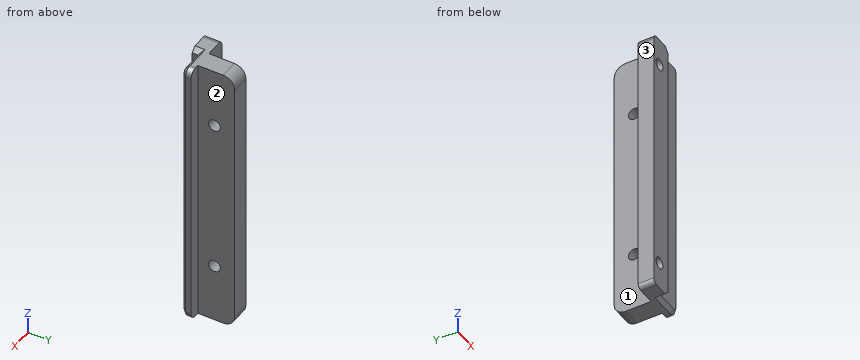
Autodesk Inventor part; units mm, degrees
ref_plane "YZ Plane" through (0, 0, 0) normal (1, 0, 0) x (0, 1, 0)
ref_plane "XZ Plane" through (0, 0, 0) normal (0, 1, 0) x (-1, 0, 0)
ref_plane "XY Plane" through (0, 0, 0) normal (0, 0, 1) x (1, 0, 0)
sketch "Sketch1" plane through (0, 0, 0) normal (0, 0, 1) x (1, 0, 0)
  line L0 (0, 17.3736) -> (0, -2.8956)
  line L1 (-5.334, 0) -> (14.224, 0)
  line L2 (3.81, 1.778) -> (-2.54, 1.778)
  line L3 (-2.54, 1.778) -> (-2.54, 0)
  line L4 (-2.54, 0) -> (3.81, 0)
  line L5 (3.81, 0) -> (3.81, 1.778)
  line L6 (3.81, 1.778) -> (11.43, 1.778)
  line L7 (11.43, 1.778) -> (11.43, 4.318)
  line L8 (11.43, 4.318) -> (-2.54, 4.318)
  line L9 (-2.54, 4.318) -> (-2.54, 1.778)
  line L10 (8.382, 4.318) -> (3.302, 4.318)
  line L11 (3.302, 4.318) -> (3.302, 14.478)
  line L12 (3.302, 14.478) -> (8.382, 14.478)
  line L13 (8.382, 14.478) -> (8.382, 4.318)
  point P0 (0, 0)
  point P1 (0, 0.635)
  dimension "d1" = 2.54
  dimension "d2" = 1.778
  dimension "d25" = 2.54
  dimension "d26" = 10.16
  dimension "d27" = 5.08
  dimension "d49" = 3.302
  dimension "d50" = 2.54
  dimension "d51" = 11.43
  dimension "d52" = 3.81
extrude "Extrusion1" add sketch "Sketch1" along normal mid plane 76.2
sketch "Sketch2" plane through (-2.54, 4.318, 38.1) normal (0, 1, 0) x (1, 0, 0)
  line L0 (13.97, 76.2) -> (13.97, 0)
  line L1 (0, 76.2) -> (13.97, 76.2)
  line L2 (13.97, 0) -> (0, 0)
  line L3 (0, 76.2) -> (0, 0)
  line L4 (16.764, 38.1) -> (-2.794, 38.1)
  point P0 (2.54, 38.1)
  point P1 (2.54, 68.58)
  point P2 (2.54, 38.1)
  point P3 (2.54, 7.62)
  dimension "d6" = 30.48
  dimension "d7" = 30.48
  dimension "d48" = 2.54
hole "Hole1" at (0, 4.318, -30.48) at (0, 4.318, 30.48) direction (0, -1, 0) diameter 3.175 end through all
fillet "Fillet4" radius 1.905 2 edges at (11.43, 3.048, 38.1) (11.43, 3.048, -38.1)
chamfer "Chamfer4" distance 1.016 angle 45 5 edges at (11.43, 1.778, 0) (10.872, 1.778, 37.542) (6.6675, 1.778, 38.1) (10.872, 1.778, -37.542) (6.6675, 1.778, -38.1)
chamfer "Chamfer1" distance 1.27 angle 45 2 edges at (3.81, 0.889, 38.1) (3.81, 0.889, -38.1)
fillet "Fillet3" radius 1.27 2 edges at (-2.54, 2.159, -38.1) (-2.54, 2.159, 38.1)
fillet "Fillet5" radius 3.175 2 edges at (5.842, 14.478, 38.1) (5.842, 14.478, -38.1)
sketch "Sketch3" plane through (8.382, 4.318, 38.1) normal (1, 0, 0) x (0, 0, -1)
  line L0 (74.93, -4.318) -> (1.27, -4.318)
  line L1 (38.1, -7.2136) -> (38.1, 13.0556)
  point P0 (38.1, -4.318)
  point P1 (16.51, 4.572)
  point P2 (59.69, 4.572)
  dimension "d38" = 43.18
  dimension "d39" = 21.59
  dimension "d40" = 8.89
hole "Hole2" at (8.382, 8.89, 21.59) at (8.382, 8.89, -21.59) direction (-1, 0, 0) diameter 3.302 end through all
properties part number "J007812" material "VERO BLACK"
Geometry: final body of the model. Coordinates: model frame, mm. Face numbers are marked on the shaded views. A direction names the side the tool comes from. Round coordinates to 2 decimals unless told otherwise and drop trailing zeros. Write each loop counter-clockwise with the first axis right and the second up, starting at its lowest first coordinate (ties: lowest second). Pieces come first, ordered by that corner, then holes.
Item 1: Section query A-A (y = 8.89). Return loops of the section in (x, z), plus the area to 3 significant figures.
Item 2: Pin query (flat end, axial travel): P1, Ø5, axis at y = 10, z = -8, coming from the +X side; P2, Ø4, axis at x = 0, z = -30.48, coming from the +Y side; P3, Ø5, axis at y = 8, z = -12, coming from the -X side; P4, Ø1.9, axis at x = 0, z = 30.48, coming from the -Y side. Return the tip coordinate at first contact, or that it passes through.
Item 3: Section query C-C (z = -21.59). Return loops of the section in (x, y), plus the area to 3 significant figures.
Item 4: Section query D-D (x = 6). Return loops of the section in (y, z) (3 decimals).
Item 5: Set-up query: the marked faces 1, 2 and 3. Return all of +Z, -Z, +X, -X, +Y, -Y with unobstructed straight access to the full face (end or side cutting, diameter ignored); none if empty.
Item 6: Section query B-B (x = 0). Return loops of the section in (y, z).
Item 7: Material intervals for L1, parallel to Z at x = 0, y = 3; L2, parallel to Z at x = 5.25, y = 8.89; L3, parallel to Y at x = 5.9, z = 21.59, sorted ascending.
Completed:
1. outline: (3.3, -38.1) - (8.38, -38.1) - (8.38, -23.24) - (3.3, -23.24) - close; (3.3, -19.94) - (8.38, -19.94) - (8.38, 19.94) - (3.3, 19.94) - close; (3.3, 23.24) - (8.38, 23.24) - (8.38, 38.1) - (3.3, 38.1) - close
1. area: 354 mm2
2. P1: stops at x = 8.38
2. P2: stops at y = 4.32
2. P3: stops at x = 3.3
2. P4: passes through
3. outline: (-2.54, 0) - (3.81, 0) - (3.81, 1.78) - (10.41, 1.78) - (11.43, 2.79) - (11.43, 4.32) - (8.38, 4.32) - (8.38, 7.24) - (3.3, 7.24) - (3.3, 4.32) - (-2.54, 4.32) - close; (3.3, 10.54) - (8.38, 10.54) - (8.38, 14.48) - (3.3, 14.48) - close
3. area: 81.1 mm2
4. outline: (1.778, -37.084) - (2.794, -38.1) - (11.303, -38.1) arc R3.175 ccw to (14.478, -34.925) - (14.478, 34.925) arc R3.175 ccw to (11.303, 38.1) - (2.794, 38.1) - (1.778, 37.084) - close; hole circle Ø3.302 at (8.89, -21.59); hole circle Ø3.302 at (8.89, 21.59)
5. face 1: +Z, -Z, -X, +Y
5. face 2: +Z, -Z, +X, +Y
5. face 3: +Z, -Z, -X, +Y, -Y
6. outline: (0, -38.1) - (4.32, -38.1) - (4.32, -32.07) - (0, -32.07) - close; (0, -28.89) - (4.32, -28.89) - (4.32, 28.89) - (0, 28.89) - close; (0, 32.07) - (4.32, 32.07) - (4.32, 38.1) - (0, 38.1) - close
7. L1: z = -38.1 to -32.07, -28.89 to 28.89, 32.07 to 38.1
7. L2: z = -38.1 to -23.24, -19.94 to 19.94, 23.24 to 38.1
7. L3: y = 1.78 to 7.24, 10.54 to 14.48
